Source: CAD feature listing. Evaluate the final solid. Frame: model axes, mm. Give positions to 0.01 mm unless a question says otherwise; leave off trailing zeros. Order: outer loops, then holes, each group sorted by start corner. A loop starts at its lowest first (then second) coordinate and runs counter-clockwise, first axis right, second up. Notation, with made-up numbers: M 23,75 L 49,75 A30 ccw 49,114 Z; hole C 9.5,54 d5. An arc over 180 degrees is marked long. Use CSV: the item, a comma, the result in double quotes. Start each with the question number.
Item 1: Section query B-B on y = 1.5. Count the separate pieces of the cut face and the enclosed holes in it, and give its area (3 significant figures).
Item 2: Section query A-A on z = -48. Return loops of the section in (x, y) (3 decimals), and give its area (3 significant figures).
Item 3: First-contact query: pin 1 (5 mm diameter, centred on x = 44.5, z = -107.5, fed in from -Y); pin 2 (1.5 mm diameter, centred on y = 1.5, z = -99, fed in from +X) (3 decimals); pin 3 (3 mm diameter, centred on x = -0.5, y = 2, fed in from -Z); pin 4 (4.5 mm diameter, centred on x = 136.52, z = -70.38, fed in from -Y). Flat tips, straight axial feed; report the tip coordinate or a pass-through.
Item 4: Ray query, probe 1 along Z at (x, y) = (9.5, 6); probe 2 along X at (y, z) = (4.75, -71) (3 decimals); probe 3 along X at (y, z) = (2, -56) (3 decimals). Return the intervals inside material, ascending. Write a range as from..to.
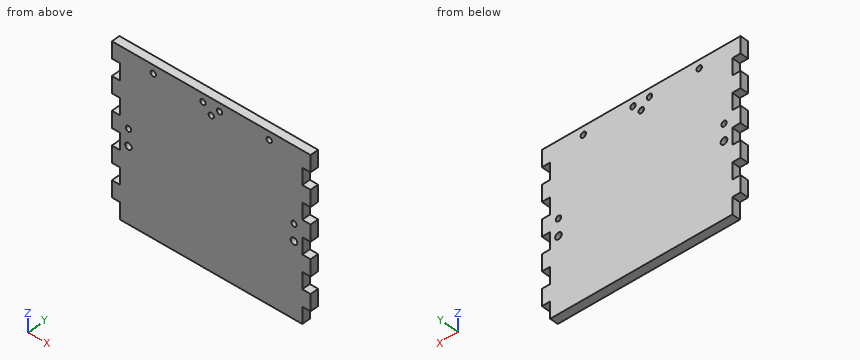
from build123d import *

# Parameters (mm, degrees)
SKETCH2_R           = 2.0828
SKETCH2_R_2         = 2.54
BOSS_EXTRUDE1_DEPTH = 6.35


with BuildPart() as part:
    # Sketch2 → Boss-Extrude1 (new body)
    with BuildSketch(Plane(origin=(0, 0, 0), x_dir=(1, 0, 0), z_dir=(0, 1, 0))):
        Polygon((3.175, 13.229166667), (3.175, 25.929166667), (-3.175, 25.929166667), (-3.175, 38.629166667), (3.175, 38.629166667), (3.175, 51.329166667), (-3.175, 51.329166667), (-3.175, 64.029166667), (3.175, 64.029166667), (3.175, 76.729166667), (-3.175, 76.729166667), (-3.175, 89.429166667), (3.175, 89.429166667), (3.175, 102.129166667), (-3.175, 102.129166667), (-3.175, 114.829166667), (3.175, 114.829166667), (3.175, 127.529166667), (142.875, 127.529166667), (142.875, 114.829166667), (149.225, 114.829166667), (149.225, 102.129166667), (142.875, 102.129166667), (142.875, 89.429166667), (149.225, 89.429166667), (149.225, 76.729166667), (142.875, 76.729166667), (142.875, 64.029166667), (149.225, 64.029166667), (149.225, 51.329166667), (142.875, 51.329166667), (142.875, 38.629166667), (149.225, 38.629166667), (149.225, 25.929166667), (142.875, 25.929166667), (142.875, 13.229166667), (149.225, 13.229166667), (149.225, 0.529166667), (-3.175, 0.529166667), (-3.175, 13.229166667), align=None)
        with Locations(Location((136.525, 57.679166667, 0), (0, 0, 90))):
            Circle(SKETCH2_R, mode=Mode.SUBTRACT)
        with Locations(Location((28.575, 6.879166667, 0), (0, 0, 270))):
            Circle(SKETCH2_R, mode=Mode.SUBTRACT)
        with Locations(Location((9.525, 57.679166667, 0), (0, 0, 270))):
            Circle(SKETCH2_R, mode=Mode.SUBTRACT)
        with Locations(Location((117.475, 6.879166667, 0), (0, 0, 90))):
            Circle(SKETCH2_R, mode=Mode.SUBTRACT)
        with Locations(Location((79.375, 6.879166667, 0), (0, 0, 270))):
            Circle(SKETCH2_R, mode=Mode.SUBTRACT)
        with Locations(Location((73.025, 13.229166667, 0), (0, 0, 270))):
            Circle(SKETCH2_R, mode=Mode.SUBTRACT)
        with Locations(Location((66.675, 6.879166667, 0), (0, 0, 270))):
            Circle(SKETCH2_R, mode=Mode.SUBTRACT)
        with Locations(Location((9.525, 70.379166667, 0), (0, 0, 270))):
            Circle(SKETCH2_R_2, mode=Mode.SUBTRACT)
        with Locations(Location((136.525, 70.379166667, 0), (0, 0, 90))):
            Circle(SKETCH2_R_2, mode=Mode.SUBTRACT)
    extrude(amount=BOSS_EXTRUDE1_DEPTH)


solid = part.part
Verdict:
1,separate pieces,"1"
1,enclosed holes,"9"
1,area,"18,400 mm2"
2,outline,"M 3.175,0 L 142.875,0 L 142.875,6.35 L 3.175,6.35 Z"
2,area,"887 mm2"
3,pin 1,"y = 0"
3,pin 2,"x = 142.875"
3,pin 3,"z = -114.83"
3,pin 4,"through"
4,probe 1,"-127.53..-72.92, -67.84..-59.76, -55.6..-0.53"
4,probe 2,"3.175..7.062, 11.988..134.062, 138.988..142.875"
4,probe 3,"-3.175..8.293, 10.757..135.293, 137.757..149.225"
